Drawing for the job (mm, zero at the part's lowest x, y, z). Give positions to 0.01 mm unless a question says otherwise; leave off trailing zeros. Order: outer loops, then holes, each group sorted by start corner. A loop starts at its lowest first (then second) coordinate and runs counter-clockwise, first axis right, second up. Notation, with made-up numbers: (22.25, 33.25) -> (59.25, 33.25) arc R31 cw to (59.25, 57.25) -> close; hole circle Ø6 at (10.25, 21.5). An arc over 180 degrees is marked (long way). Use one line per item in the form item = value. Start each with the question number.
1) Drop a flat-ended pin along its axis: P1, Ø4, axis at x = 9.46, y = 15.59, coming from the +Z side. Give the stop position or say it passes through.
2) Probe line 1 (Y direction, x = 9.5, z = 4.45) (1 decimal); line 2 (X direction, y = 89, z = 0.3) (1 decimal); line 3 (Y direction, x = 94, z = 3.1). List the from-to ranges inside material, lowest first.
3) Cut at A-A, the plane y = 88. Give the cut face in (x, z), and give its area (3 significant figures).
4) Cut at B-B, the plane z = 3.6. State how many separate pieces and enclosed holes the cut face has, and give its area (3 significant figures).
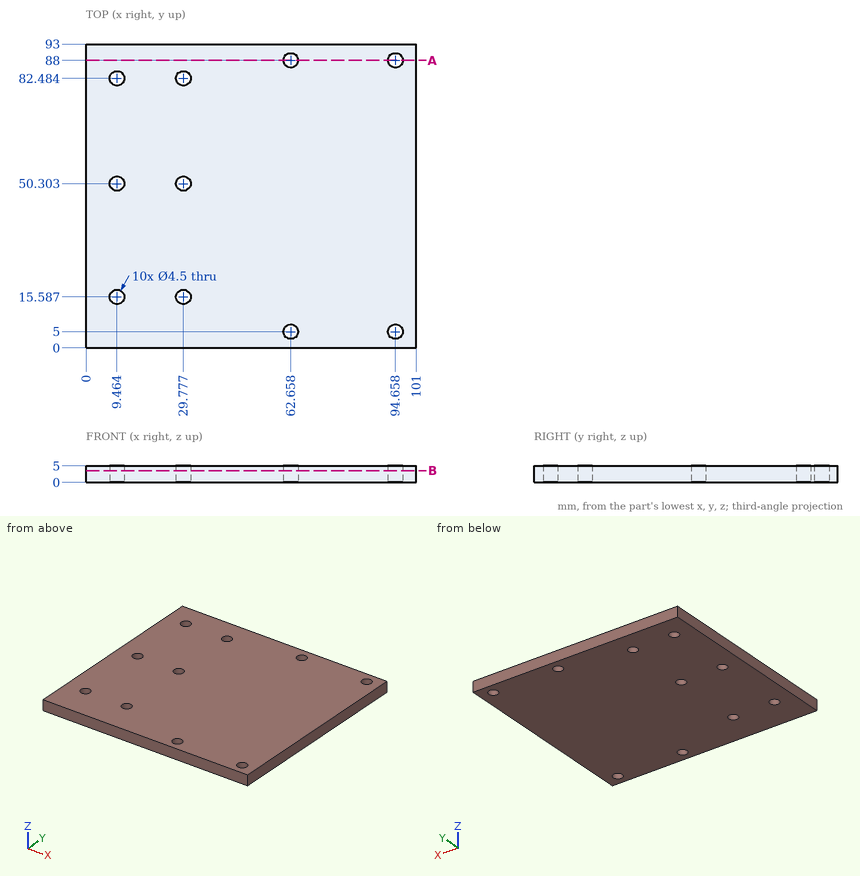
Result:
q1.P1 = through
q2.line_1 = 0 to 13.3, 17.8 to 48.1, 52.6 to 80.2, 84.7 to 93
q2.line_2 = 0 to 60.6, 64.7 to 92.6, 96.7 to 101
q2.line_3 = 0 to 2.85, 7.15 to 85.85, 90.15 to 93
q3.outline = (0, 0) -> (60.41, 0) -> (60.41, 5) -> (0, 5) -> close; (64.91, 0) -> (92.41, 0) -> (92.41, 5) -> (64.91, 5) -> close; (96.91, 0) -> (101, 0) -> (101, 5) -> (96.91, 5) -> close
q3.area = 460 mm²
q4.separate_pieces = 1
q4.enclosed_holes = 10
q4.area = 9,230 mm²
